from build123d import *

# Parameters (mm, degrees)
PAD_DEPTH       = 34
SKETCH001_R     = 18
PAD001_DEPTH    = 20
SKETCH002_W     = 100
SKETCH002_H     = 100
PAD002_DEPTH    = 20
SKETCH003_R     = 50
PAD003_DEPTH    = 20
CHAMFER_SIZE    = 2
SKETCH004_R     = 20
POCKET_DEPTH    = 20
SKETCH005_W     = 96
SKETCH005_H     = 10
POCKET001_DEPTH = 16
SKETCH006_W     = 10
SKETCH006_H     = 100
POCKET002_DEPTH = 2


with BuildPart() as part:
    # Sketch → Pad (new body, symmetric)
    with BuildSketch(Plane.XZ):
        with BuildLine():
            ThreePointArc((-48, 0), (0, -48), (48, 0))
            Line((48, 50), (48, 0))
            Line((-48, 50), (48, 50))
            Line((-48, 0), (-48, 50))
        make_face()
    extrude(amount=PAD_DEPTH, both=True)

    # Sketch001 (on Face6 of Pad) → Pad001 (join)
    with BuildSketch(Plane.XZ.offset(34)):
        Circle(SKETCH001_R)
    pad001 = extrude(amount=PAD001_DEPTH)

    # Mirrored: Pad001 across XZ
    add(pad001.mirror(Plane.XZ))

    # Sketch002 (on Face6 of Mirrored) → Pad002 (join)
    with BuildSketch(Plane(origin=(0, 0, 50), x_dir=(-1, 0, 0), z_dir=(0, 0, 1))):
        Rectangle(SKETCH002_W, SKETCH002_H)
    extrude(amount=PAD002_DEPTH)

    # Sketch003 (on Face5 of Pad002) → Pad003 (join)
    with BuildSketch(Plane(origin=(0, 0, 70), x_dir=(-1, 0, 0), z_dir=(0, 0, 1))):
        Circle(SKETCH003_R)
    extrude(amount=PAD003_DEPTH)

    # Chamfer
    chamfer_edges = [part.edges().sort_by_distance(p)[0] for p in [
        (50, 0, 90),
    ]]
    chamfer(chamfer_edges, length=CHAMFER_SIZE)

    # Sketch004 (on Face7 of Chamfer) → Pocket (cut)
    with BuildSketch(Plane(origin=(0, 0, 90), x_dir=(-1, 0, 0), z_dir=(0, 0, 1))):
        Circle(SKETCH004_R)
    extrude(amount=-POCKET_DEPTH, mode=Mode.SUBTRACT)

    # Sketch005 (on Face11 of Pocket) → Pocket001 (cut)
    with BuildSketch(Plane.XZ.offset(50)):
        with Locations((0, 55)):
            Rectangle(SKETCH005_W, SKETCH005_H)
    pocket001 = extrude(amount=-POCKET001_DEPTH, mode=Mode.SUBTRACT)

    # Mirrored001: Pocket001 across XZ
    add(pocket001.mirror(Plane.XZ), mode=Mode.SUBTRACT)

    # Sketch006 (on Face10 of Mirrored001) → Pocket002 (cut)
    with BuildSketch(Plane(origin=(50, 0, 0), x_dir=(0, 0, 1), z_dir=(1, 0, 0))):
        with Locations((55, 0)):
            Rectangle(SKETCH006_W, SKETCH006_H)
    pocket002 = extrude(amount=-POCKET002_DEPTH, mode=Mode.SUBTRACT)

    # Mirrored002: Pocket002 across YZ
    add(pocket002.mirror(Plane.YZ), mode=Mode.SUBTRACT)


solid = part.part
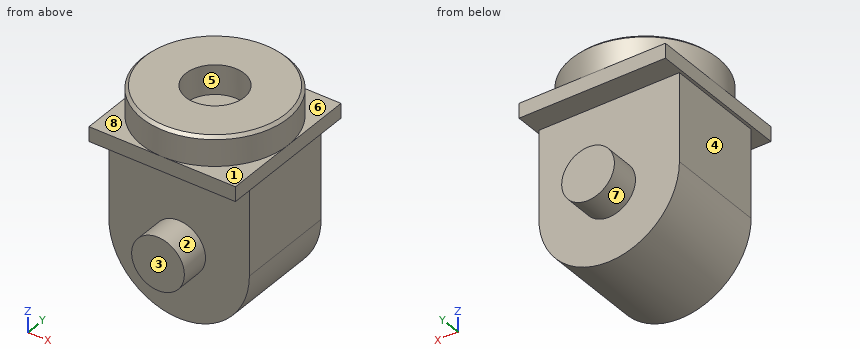
The listing builds one solid part. Answer for the finished solid, in the listing's coordinates (mm). Face numbers are marked on the shaded views. A direction names the side the tool comes from. Round coordinates to 2 decimals unless told otherwise and drop trailing zeros. Write each loop counter-clockwise with the first axis right and the second up, starting at its lowest first coordinate (ties: lowest second). Pieces come first, ordered by that corner, then holes. Notation, with made-up numbers: M 52.25,55.5 L 104.25,55.5 A12 ccw 104.25,67.5 Z; hole C -29,-38.75 d11. An arc over 180 degrees is marked long. Write each question's results on one line, items separated by ' | '. Start each with the question number.
Item 1: Given pin 1 Ø11 at (x, z) = (16, 67) entering from -Y; pin 2 Ø6 at (x, y) = (3, 2) entering from -Z; pin 3 Ø2 at (y, z) = (-1.5, 49) entering from +X, each flat-ended and moving along its own axis, determine where each tip first touches the part or whether it passes through.
Item 2: The mould has two halves that part along Z. Classify the marked faces 1, 2 and 3: +Z half, -Z half, draft (parallel to the pull), parting line (faces both ways), or undercut.
Item 3: Which of the six approach directions +Z, -Z, +X, -X, +Y, -Y give full straight-line access (tool end or side, diameter ignored) to the marked faces 4, 5, 6, 7 and 8?
Item 4: Find section B-B on z = 39.5. Write down the section's boundary in (x, y).
Item 5: Find section A-A on z = -15. Write down the section's boundary in (x, y).
Item 6: Find section C-C on z = 2. Write down the section's boundary in (x, y), and give its area (3 significant figures).
Item 7: Straight lines are drawn through the part: probe 1 along X at (y, z) = (0, 74); probe 2 along Y at (x, z) = (-33, -28). For each, find the intervals that lie inside material, in ascending order.
Item 8: Find section D-D on z = 62.5. Write down the section's boundary in (x, y), and give its area (3 significant figures).
Answer block:
1) pin 1: stops at y = -50 | pin 2: stops at z = -48 | pin 3: stops at x = 48
2) face 1: +Z half | face 2: undercut | face 3: draft
3) face 4: -Z, -X, +Y, -Y | face 5: +Z | face 6: +Z, +X, +Y | face 7: +Y | face 8: +Z, -X, -Y
4) outline: M -48,-34 L 48,-34 L 48,34 L -48,34 Z
5) outline: M -45.6,-34 L -9.95,-34 L -9.95,-54 L 9.95,-54 L 9.95,-34 L 45.6,-34 L 45.6,34 L 9.95,34 L 9.95,54 L -9.95,54 L -9.95,34 L -45.6,34 Z
6) outline: M -48,-34 L -17.89,-34 L -17.89,-54 L 17.89,-54 L 17.89,-34 L 48,-34 L 48,34 L 17.89,34 L 17.89,54 L -17.89,54 L -17.89,34 L -48,34 Z | area: 7,960 mm²
7) probe 1: x = -50 to -20, 20 to 50 | probe 2: y = -34 to 34
8) outline: M -50,-50 L 50,-50 L 50,50 L -50,50 Z | area: 10,000 mm²
